Input: dimensioned drawing with shaded views. Units: mm. Origin: part minimum x, y, z. A direction names the side the tool comes from. Round coordinates to 2 decimals unless told otherwise and drop trailing zeros. Loops run counter-clockwise (first coordinate to the right, second up) from the corner with the lowest first, then second, coordinate; pieces in that order, holes last.
1) Section D-D, the plane z = 53. Return loops of the section in (x, y), and give its area (3 significant figures).
2) Access query for the marked faces 1 and 2. Directions: +Z, -Z, +X, -X, +Y, -Y. A direction counts if a zero-diameter tool reaches every point of the face in a straight line with its end or side. Return the directions, or none.
3) First-contact query: pin 1 (3 mm diameter, centred on y = 12.5, z = 15.5, fed in from +X); pin 2 (6 mm diameter, centred on x = 23, y = 9, fed in from +Z); pin 3 (12 mm diameter, centred on y = 27, z = 62.5, fed in from +X). Flat tips, straight axial feed; report the tip coordinate or a pass-through.
4) Section C-C, the plane y = 34.5. Return loops of the section in (x, z), and give its area (3 significant figures).
5) Section B-B, the plane x = 28.5. Return loops of the section in (y, z).
6) Ray query, line 1 along Z through (x, y) = (24.5, 35.5); line 2 along X through (y, z) = (3, 9); line 3 along X through (y, z) = (4, 42). Return the intervals inside material, ascending.
7) Section A-A, the plane z = 34. Return loops of the section in (x, y), and give its area (3 significant figures).
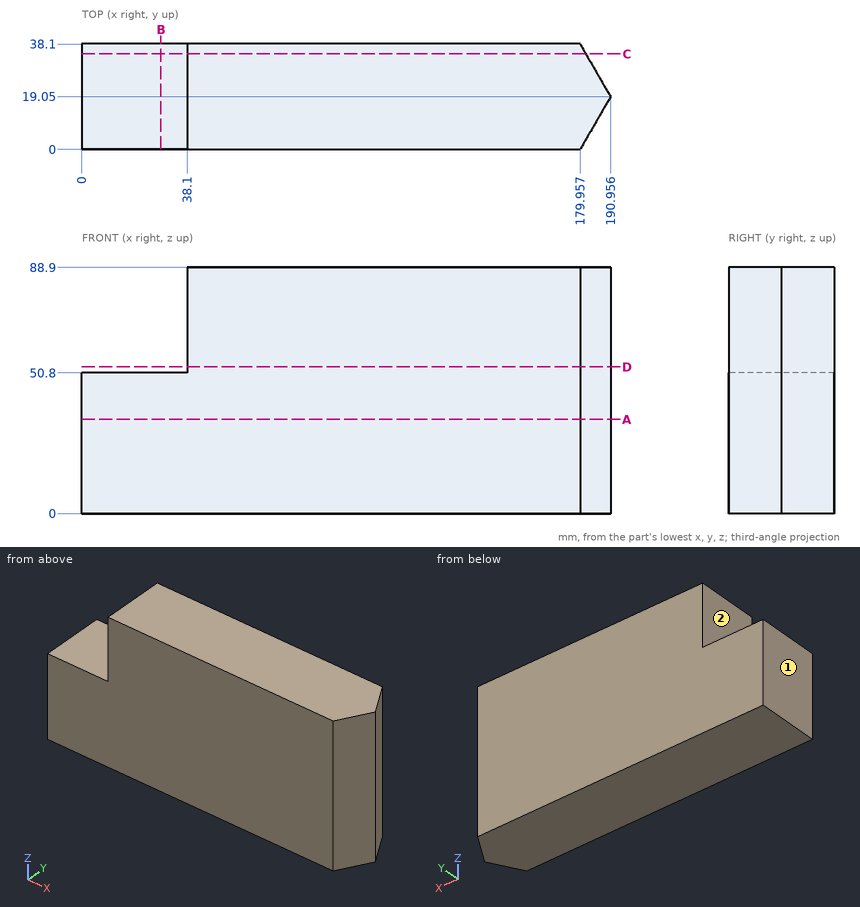
Final values:
1. outline: (38.1, 0) - (179.96, 0) - (190.96, 19.05) - (179.96, 38.1) - (38.1, 38.1) - close
1. area: 5,610 mm2
2. face 1: +Z, -Z, -X, +Y, -Y
2. face 2: +Z, -X, +Y, -Y
3. pin 1: stops at x = 188.04
3. pin 2: stops at z = 50.8
3. pin 3: stops at x = 189.83
4. outline: (0, 0) - (182.04, 0) - (182.04, 88.9) - (38.1, 88.9) - (38.1, 50.8) - (0, 50.8) - close
4. area: 14,700 mm2
5. outline: (0, 0) - (38.1, 0) - (38.1, 50.8) - (0, 50.8) - close
6. line 1: z = 0 to 50.8
6. line 2: x = 0 to 181.69
6. line 3: x = 0 to 182.27
7. outline: (0, 0) - (179.96, 0) - (190.96, 19.05) - (179.96, 38.1) - (0, 38.1) - close
7. area: 7,070 mm2
